Source: CAD feature listing. Evaluate the final solid. Frame: model axes, mm. Give positions to 0.01 mm unless a question says otherwise; leave off trailing zeros. Write each loop counter-clockwise with the first axis right and the second up, starting at its lowest first coordinate (ties: lowest second). Pieces come first, ordered by that corner, then holes. Notation, with made-up numbers: M 38,35 L 68,35 A18 ccw 68,61 Z; hole C 46.25,-1 d8. An arc over 180 degrees is marked long. Return JSON: item names as keys, results as strings.
```python
from build123d import *

# Parameters (mm, degrees)
Y_KSEKLIK_EKSTR_ZYON1_DEPTH = 2
IZIM2_R                     = 19.3
KES_EKSTR_ZYON1_DEPTH       = 3
IZIM3_R                     = 1
KES_EKSTR_ZYON2_DEPTH       = 3
IZIM4_R                     = 1
KES_EKSTR_ZYON3_DEPTH       = 3


with BuildPart() as part:
    # Çizim1 → Yükseklik-Ekstrüzyon1 (new body)
    with BuildSketch(Plane.XY):
        with BuildLine():
            Line((-11.113505298, 25.7), (11.113505298, 25.7))
            ThreePointArc((11.113505298, 25.7), (28, 0), (11.113505298, -25.7))
            Line((11.113505298, -25.7), (-11.113505298, -25.7))
            ThreePointArc((-11.113505298, -25.7), (-28, 0), (-11.113505298, 25.7))
        make_face()
    extrude(amount=Y_KSEKLIK_EKSTR_ZYON1_DEPTH)

    # Çizim2 → Kes-Ekstrüzyon1 (cut)
    with BuildSketch(Plane.XY.offset(2)):
        Circle(IZIM2_R)
    extrude(amount=-KES_EKSTR_ZYON1_DEPTH, mode=Mode.SUBTRACT)

    # Çizim3 → Kes-Ekstrüzyon2 (cut)
    with BuildSketch(Plane.XY.offset(2)):
        with Locations((-23, 0)):
            Circle(IZIM3_R)
        with Locations((-22.776165581, 3.200981322)):
            Circle(IZIM3_R)
        with Locations((-22.109019007, 6.339659184)):
            Circle(IZIM3_R)
        with Locations((-21.011545526, 9.354942791)):
            Circle(IZIM3_R)
        with Locations((-19.505106212, 12.188143077)):
            Circle(IZIM3_R)
        with Locations((-17.619022192, 14.784115023)):
            Circle(IZIM3_R)
        with Locations((-15.390003946, 17.092330986)):
            Circle(IZIM3_R)
        with Locations((-12.86143678, 19.067864169)):
            Circle(IZIM3_R)
        with Locations((-10.082536376, 20.672263065)):
            Circle(IZIM3_R)
        with Locations((-10.082536376, -20.672263065)):
            Circle(IZIM3_R)
        with Locations((-12.86143678, -19.067864169)):
            Circle(IZIM3_R)
        with Locations((-15.390003946, -17.092330986)):
            Circle(IZIM3_R)
        with Locations((-17.619022192, -14.784115023)):
            Circle(IZIM3_R)
        with Locations((-19.505106212, -12.188143077)):
            Circle(IZIM3_R)
        with Locations((-21.011545526, -9.354942791)):
            Circle(IZIM3_R)
        with Locations((-22.109019007, -6.339659184)):
            Circle(IZIM3_R)
        with Locations((-22.776165581, -3.200981322)):
            Circle(IZIM3_R)
        with Locations((10.082536376, -20.672263065)):
            Circle(IZIM3_R)
        with Locations((12.86143678, -19.067864169)):
            Circle(IZIM3_R)
        with Locations((15.390003946, -17.092330986)):
            Circle(IZIM3_R)
        with Locations((17.619022192, -14.784115023)):
            Circle(IZIM3_R)
        with Locations((19.505106212, -12.188143077)):
            Circle(IZIM3_R)
        with Locations((21.011545526, -9.354942791)):
            Circle(IZIM3_R)
        with Locations((22.109019007, -6.339659184)):
            Circle(IZIM3_R)
        with Locations((22.776165581, -3.200981322)):
            Circle(IZIM3_R)
        with Locations((23, 0)):
            Circle(IZIM3_R)
        with Locations((22.776165581, 3.200981322)):
            Circle(IZIM3_R)
        with Locations((22.109019007, 6.339659184)):
            Circle(IZIM3_R)
        with Locations((21.011545526, 9.354942791)):
            Circle(IZIM3_R)
        with Locations((19.505106212, 12.188143077)):
            Circle(IZIM3_R)
        with Locations((17.619022192, 14.784115023)):
            Circle(IZIM3_R)
        with Locations((15.390003946, 17.092330986)):
            Circle(IZIM3_R)
        with Locations((12.86143678, 19.067864169)):
            Circle(IZIM3_R)
        with Locations((10.082536376, 20.672263065)):
            Circle(IZIM3_R)
    extrude(amount=-KES_EKSTR_ZYON2_DEPTH, mode=Mode.SUBTRACT)

    # Çizim4 → Kes-Ekstrüzyon3 (cut)
    with BuildSketch(Plane.XY.offset(2)):
        with Locations((-12.20385672, 22.793583408)):
            Circle(IZIM4_R)
        with Locations((-12.577279495, -22.589679146)):
            Circle(IZIM4_R)
        with Locations((-15.664107459, -20.569815287)):
            Circle(IZIM4_R)
        with Locations((-18.432059367, -18.131209307)):
            Circle(IZIM4_R)
        with Locations((-20.8247877, -15.323504191)):
            Circle(IZIM4_R)
        with Locations((-22.793583408, -12.20385672)):
            Circle(IZIM4_R)
        with Locations((-24.29836749, -8.835773918)):
            Circle(IZIM4_R)
        with Locations((-25.308506881, -5.28782024)):
            Circle(IZIM4_R)
        with Locations((-25.803438055, -1.632221791)):
            Circle(IZIM4_R)
        with Locations((-25.773085641, 2.056603987)):
            Circle(IZIM4_R)
        with Locations((-25.218067527, 5.703563239)):
            Circle(IZIM4_R)
        with Locations((-24.149682281, 9.234414391)):
            Circle(IZIM4_R)
        with Locations((-22.589679146, 12.577279495)):
            Circle(IZIM4_R)
        with Locations((-20.569815287, 15.664107459)):
            Circle(IZIM4_R)
        with Locations((-18.131209307, 18.432059367)):
            Circle(IZIM4_R)
        with Locations((-15.323504191, 20.8247877)):
            Circle(IZIM4_R)
        with Locations((12.577279495, -22.589679146)):
            Circle(IZIM4_R)
        with Locations((15.664107459, -20.569815287)):
            Circle(IZIM4_R)
        with Locations((18.432059367, -18.131209307)):
            Circle(IZIM4_R)
        with Locations((20.8247877, -15.323504191)):
            Circle(IZIM4_R)
        with Locations((22.793583408, -12.20385672)):
            Circle(IZIM4_R)
        with Locations((24.29836749, -8.835773918)):
            Circle(IZIM4_R)
        with Locations((25.308506881, -5.28782024)):
            Circle(IZIM4_R)
        with Locations((25.803438055, -1.632221791)):
            Circle(IZIM4_R)
        with Locations((25.773085641, 2.056603987)):
            Circle(IZIM4_R)
        with Locations((25.218067527, 5.703563239)):
            Circle(IZIM4_R)
        with Locations((24.149682281, 9.234414391)):
            Circle(IZIM4_R)
        with Locations((22.589679146, 12.577279495)):
            Circle(IZIM4_R)
        with Locations((20.569815287, 15.664107459)):
            Circle(IZIM4_R)
        with Locations((18.131209307, 18.432059367)):
            Circle(IZIM4_R)
        with Locations((15.323504191, 20.8247877)):
            Circle(IZIM4_R)
        with Locations((12.20385672, 22.793583408)):
            Circle(IZIM4_R)
    extrude(amount=-KES_EKSTR_ZYON3_DEPTH, mode=Mode.SUBTRACT)


solid = part.part
```
1) Line query: line 1 (Y direction, x = -14.5, z = 1.4); line 2 (Y direction, x = 11.5, z = 0.4); line 3 (X direction, y = 12, z = 1.8). Output: solid intervals per line, ascending. Write a range as [from, to].
Numbers:
{"line 1": "y = [-23.95, -17.55], [-16.64, -12.74], [12.74, 16.64], [17.55, 20.26], [21.39, 23.95]", "line 2": "y = [-25.53, -15.5], [15.5, 22.08], [23.5, 25.53]", "line 3": "x = [-25.3, -23.41], [-21.77, -20.49], [-18.52, -15.12], [15.12, 18.52], [20.49, 21.77], [23.41, 25.3]"}
2) Draft query along X for faces 1 (the face through (28, 0, 1)), 2 (the face through (20.43, -12.57, 1.01)), 3 (the face through (11.784, -23.198, 1.014)). Return one class per face: released by +X, released by -X, zero draft, split by the parting line, or undercut.
Numbers:
{"face 1": "released by +X", "face 2": "undercut", "face 3": "undercut"}
3) Cut plane A-A, the plane x = 0. Return the cut outline in (y, z), then the cut area to 3 significant figures.
Numbers:
{"outline": "M -25.7,0 L -19.3,0 L -19.3,2 L -25.7,2 Z; M 19.3,0 L 25.7,0 L 25.7,2 L 19.3,2 Z", "area": "25.6 mm²"}
4) Cut plane D-D, the plane z = 1.25. Give the number of separate pieces and of enclosed holes in the cut face, then the cut area to 3 significant figures.
Numbers:
{"separate pieces": "1", "enclosed holes": "67", "area": "1,020 mm²"}
5) Cut plane B-B, the plane y = 0. Return the cut outline in (x, z), then the cut area to 3 significant figures.
Numbers:
{"outline": "M -28,0 L -24,0 L -24,2 L -28,2 Z; M -22,0 L -19.3,0 L -19.3,2 L -22,2 Z; M 19.3,0 L 22,0 L 22,2 L 19.3,2 Z; M 24,0 L 28,0 L 28,2 L 24,2 Z", "area": "26.8 mm²"}
6) Cut plane C-C, the plane x = -10. Return the cut outline in (y, z), then the cut area to 3 significant figures.
Numbers:
{"outline": "M -25.7,0 L -21.67,0 L -21.67,2 L -25.7,2 Z; M -19.68,0 L -16.51,0 L -16.51,2 L -19.68,2 Z; M 16.51,0 L 19.68,0 L 19.68,2 L 16.51,2 Z; M 21.67,0 L 25.7,0 L 25.7,2 L 21.67,2 Z", "area": "28.8 mm²"}
7) Contact query for flat-ended pins moving along their axis: pin 1 Ø1.2 at (x, y) = (15.32, 20.82) entering from -Z; pin 2 Ø1 at (y, z) = (9, 1.5) entering from -X. Output: stop coordinate, or through.
Numbers:
{"pin 1": "passes through", "pin 2": "stops at x = -26.68"}
